The model under review builds one solid part; all positions refer to its coordinate system, in mm. A direction names the side the tool comes from. Round coordinates to 2 decimals unless told otherwise and drop trailing zeros. Loops run counter-clockwise (first coordinate to the right, second up) from the corner with the lowest first, then second, coordinate; pieces in that order, holes last. Notation, with made-up numbers: (60.25, -1) - (103.25, -1) arc R30 cw to (103.25, 38) - close; hole circle Ø4 at (30.25, 62.5). An arc over 180 degrees is marked (long way). Answer as CSV lines item,"result".
from build123d import *

# Parameters (mm, degrees)
F2_R     = 1
F3_SIZE  = 1
F5_DEPTH = 4
F7_DEPTH = 4


with BuildPart() as f1:
    # F0 (on Front) → F1 (revolve)
    with BuildSketch(Plane.XZ):
        Polygon((-32, 14), (-32, 10), (-17, 10), (-17, 8), (18, 8), (18, 10), (33, 10), (33, 14), align=None)
    revolve(axis=Axis((4.3690800667, 0, 0), (-1, 0, 0)))

    # F2
    f2_edges = [f1.edges().sort_by_distance(p)[0] for p in [
        (18, 0, -10),
        (-17, 0, -10),
    ]]
    fillet(f2_edges, radius=F2_R)

    # F3
    f3_edges = [f1.edges().sort_by_distance(p)[0] for p in [
        (-32, 0, -10),
        (33, 0, -10),
    ]]
    chamfer(f3_edges, length=F3_SIZE)

    # F4 (on face) → F5 (cut)
    with BuildSketch(Plane(origin=(-32, 0, 0), x_dir=(0, -1, 0), z_dir=(-1, 0, 0))):
        with BuildLine():
            Line((0, 14), (-10, 14))
            Line((-10, 14), (-10, 12))
            Line((-10, 12), (-7.2111025509, 12))
            ThreePointArc((-7.2111025509, 12), (-3.7416573868, 13.4907375632), (0, 14))
        make_face()
        with BuildLine():
            ThreePointArc((7.2111025509, 12), (3.7416573868, 13.4907375632), (0, 14))
            ThreePointArc((0, 14), (-3.7416573868, 13.4907375632), (-7.2111025509, 12))
            Line((-7.2111025509, 12), (7.2111025509, 12))
        make_face()
        with BuildLine():
            Line((10, 14), (0, 14))
            ThreePointArc((0, 14), (3.7416573868, 13.4907375632), (7.2111025509, 12))
            Line((7.2111025509, 12), (10, 12))
            Line((10, 12), (10, 14))
        make_face()
        with BuildLine():
            ThreePointArc((0, -14), (-3.7416573868, -13.4907375632), (-7.2111025509, -12))
            Line((-7.2111025509, -12), (-10, -12))
            Line((-10, -12), (-10, -14))
            Line((-10, -14), (0, -14))
        make_face()
        with BuildLine():
            Line((7.2111025509, -12), (-7.2111025509, -12))
            ThreePointArc((-7.2111025509, -12), (-3.7416573868, -13.4907375632), (0, -14))
            ThreePointArc((0, -14), (3.7416573868, -13.4907375632), (7.2111025509, -12))
        make_face()
        with BuildLine():
            Line((10, -12), (7.2111025509, -12))
            ThreePointArc((7.2111025509, -12), (3.7416573868, -13.4907375632), (0, -14))
            Line((0, -14), (10, -14))
            Line((10, -14), (10, -12))
        make_face()
    extrude(amount=-F5_DEPTH, mode=Mode.SUBTRACT)

    # F6 (on face) → F7 (cut)
    with BuildSketch(Plane.YZ.offset(33)):
        with BuildLine():
            ThreePointArc((7.2111025509, 12), (3.7416573868, 13.4907375632), (0, 14))
            ThreePointArc((0, 14), (-3.7416573868, 13.4907375632), (-7.2111025509, 12))
            Line((-7.2111025509, 12), (7.2111025509, 12))
        make_face()
        with BuildLine():
            Line((7.2111025509, -12), (-7.2111025509, -12))
            ThreePointArc((-7.2111025509, -12), (-3.7416573868, -13.4907375632), (0, -14))
            ThreePointArc((0, -14), (3.7416573868, -13.4907375632), (7.2111025509, -12))
        make_face()
    extrude(amount=-F7_DEPTH, mode=Mode.SUBTRACT)


solid = f1.part
1. Take a section at B-B (z = 0). State the section outline as (x, y) points, plus the area to 3 significant figures.
Numbers:
outline,"(-32, -14) - (33, -14) - (33, -11) - (32, -10) - (19, -10) arc R1 cw to (18, -9) - (18, -8) - (-17, -8) - (-17, -9) arc R1 cw to (-18, -10) - (-31, -10) - (-32, -11) - close; (-32, 11) - (-31, 10) - (-18, 10) arc R1 cw to (-17, 9) - (-17, 8) - (18, 8) - (18, 9) arc R1 cw to (19, 10) - (32, 10) - (33, 11) - (33, 14) - (-32, 14) - close"
area,"659 mm²"
2. Take a section at D-D (x = -2.5). State the section outline as (y, z) points, plus the area to 3 significant figures.
Numbers:
outline,"circle Ø28 at (0, 0); hole circle Ø16 at (0, 0)"
area,"415 mm²"
3. Take a section at C-C (x = 27.5). State the section outline as (y, z) points.
Numbers:
outline,"circle Ø28 at (0, 0); hole circle Ø20 at (0, 0)"
4. Clearance check with flat-ended pins moving along their axes: pin 1 (1.2 mm diameter, centred on x = -29.5, y = 2.5, fed in from -Z); pin 2 (2 mm diameter, centred on x = 30.5, y = 2, fed in from +Z); pin 3 (2 mm diameter, centred on y = -9.5, z = -1, fed in from -X). State where each tip first meets the part, or that it passes through.
Numbers:
pin 1,"stops at z = -12"
pin 2,"stops at z = 12"
pin 3,"stops at x = -31.55"
5. Draft analysis for pull direction Z (two halves, no side actions). For faces 1 (the face through (-30, 0, 12)), 2 (the face through (-24.41, -9.76, -2.17)), 3 (the face through (0.75, -7.81, -1.73)), 4 (the face through (29, 0, 13)), state which applies: +Z half, -Z half, draft (parallel to the pull), parting line (faces both ways), or undercut.
Numbers:
face 1,"+Z half"
face 2,"undercut"
face 3,"undercut"
face 4,"draft"
6. Tool access review of faces 5 (the face through (31, 0, 12)), 6 (the face through (25.59, -9.76, -2.17)), 7 (the face through (-28, 0, 13)), 8 (the face through (31, 0, -12)): name each direction out of +Z, -Z, +X, -X, +Y, -Y from which nothing blocks a thin tool from reaching the whole face with its end or side.
Numbers:
face 5,"+Z, +X, +Y, -Y"
face 6,"+X"
face 7,"+Z, -X, +Y, -Y"
face 8,"-Z, +X, +Y, -Y"
7. Wall thickness on probe 1 along Y at (x, z) = (-27.5, 0); probe 2 along Y at (x, z) = (5.5, 0); probe 3 along X at (y, z) = (0.75, -12.5): over which ranges is each line inside the solid? List them lowest first.
Numbers:
probe 1,"y = -14 to -10, 10 to 14"
probe 2,"y = -14 to -8, 8 to 14"
probe 3,"x = -28 to 29"
